```python
from build123d import *

# Parameters (mm, degrees)
F0_W     = 146
F0_H     = 74
F1_DEPTH = 4
F3_DEPTH = 2
F2_W     = 6
F2_H     = 37
F4_DEPTH = 2
F5_DEPTH = 2


with BuildPart() as f1:
    # F0 (on Front) → F1 (new body)
    with BuildSketch(Plane.XZ):
        with Locations((73, 37)):
            Rectangle(F0_W, F0_H)
    extrude(amount=F1_DEPTH)

    # F2 (on face) → F3 (cut)
    with BuildSketch(Plane.XZ.offset(4)):
        Polygon((3, 3), (3, 74), (0, 74), (0, 0), (96, 0), (96, 23), (93, 23), (93, 3), align=None)
    extrude(amount=-F3_DEPTH, mode=Mode.SUBTRACT)

    # F2 (on face) → F4 (cut)
    with BuildSketch(Plane.XZ.offset(4)):
        with Locations((92, 55.5)):
            Rectangle(F2_W, F2_H)
    extrude(amount=-F4_DEPTH, mode=Mode.SUBTRACT)

    # F2 (on face) → F5 (cut)
    with BuildSketch(Plane.XZ.offset(4)):
        Polygon((93, 28), (93, 23), (96, 23), (146, 23), (146, 31), (96, 31), (96, 28), align=None)
    extrude(amount=-F5_DEPTH, mode=Mode.SUBTRACT)


solid = f1.part
```
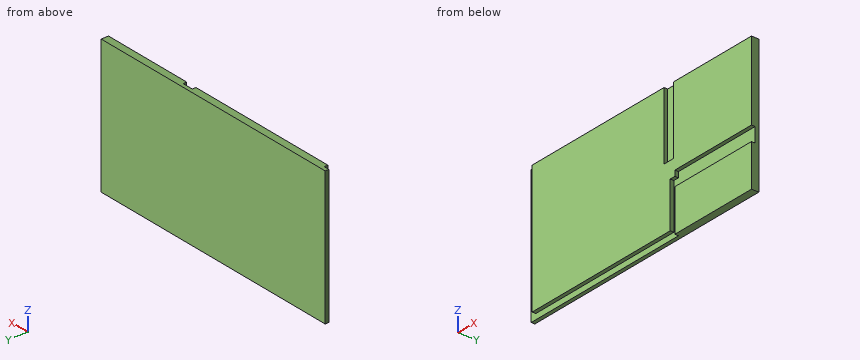
Source: CAD feature listing. Evaluate the final solid. Frame: model axes, mm. Give positions to 0.01 mm unless a question says otherwise; leave off trailing zeros. Loops run counter-clockwise (first coordinate to the right, second up) from the corner with the lowest first, then second, coordinate; pieces in that order, holes last. Notation, with made-up numbers: M 13.25,-36 L 40.25,-36 A27 ccw 40.25,-18 Z; hole C 43,-18 d8. An arc over 180 degrees is marked long. Put each result on its own line as item: value.
Q1. Section D-D (z = 43). Return the cut outline in (x, y), and give its area (3 significant figures).
Response values:
outline: M 0,-2 L 3,-2 L 3,-4 L 89,-4 L 89,-2 L 95,-2 L 95,-4 L 146,-4 L 146,0 L 0,0 Z
area: 566 mm²
Q2. Section B-B (z = 15.5). Return the cut outline in (x, y).
Response values:
outline: M 0,-2 L 3,-2 L 3,-4 L 93,-4 L 93,-2 L 96,-2 L 96,-4 L 146,-4 L 146,0 L 0,0 Z
Q3. Line query: probe 1 along Z at (x, y) = (137.5, -2.2); probe 2 along X at (y, z) = (-2.7, 44.5); probe 3 along X at (y, z) = (-2.95, 7). Output: solid intervals per line, ascending. Write a range as [from, to].
Response values:
probe 1: z = [0, 23], [31, 74]
probe 2: x = [3, 89], [95, 146]
probe 3: x = [3, 93], [96, 146]
Q4. Pin query (flat end, axial travel): P1, Ø0.6, axis at y = -3, z = 60, coming from the -X side; P2, Ø1.6, axis at x = 94, y = -3, coming from the -Z side. Return the tip coordinate at first contact, or that it passes through.
Response values:
P1: stops at x = 3
P2: stops at z = 28
Q5. Section A-A (y = -2.6). Return the cut outline in (x, z), and give its area (3 significant figures).
Response values:
outline: M 3,3 L 93,3 L 93,28 L 96,28 L 96,31 L 146,31 L 146,74 L 95,74 L 95,37 L 89,37 L 89,74 L 3,74 Z; M 96,0 L 146,0 L 146,23 L 96,23 Z
area: 9,610 mm²
Q6. Section C-C (x = 19.5). Return the cut outline in (y, z).
Response values:
outline: M -4,3 L -2,3 L -2,0 L 0,0 L 0,74 L -4,74 Z
